Design review of the part built by this model. Coordinates are the model's own, in mm. Face numbers are marked on the shaded views. A direction names the side the tool comes from. Round coordinates to 2 decimals unless told otherwise and drop trailing zeros. Write each loop counter-clockwise with the first axis right and the second up, starting at its lowest first coordinate (ties: lowest second). Pieces come first, ordered by that corner, then holes. Notation, with made-up numbers: (13.5, 16) - (32.5, 16) arc R7 cw to (32.5, 26) - close; hole circle Ø8 at (-10, -24). An arc over 180 degrees is marked (long way). Use one line per item in the form item = value.
```python
from build123d import *

# Parameters (mm, degrees)
SKETCH1_W           = 2.8702
SKETCH1_H           = 3.5052
SKETCH2_R           = 1.7526
BOSS_EXTRUDE1_DEPTH = 7.9375
CUT_EXTRUDE1_DEPTH  = 1.6256
CHAMFER1_SIZE       = 0.47244
CHAMFER2_SIZE       = 0.3556
FILLET1_R           = 0.254


with BuildPart() as part:
    # Sketch1 → Revolve1 (revolve)
    with BuildSketch(Plane.XY):
        with Locations((1.4351, 1.7526)):
            Rectangle(SKETCH1_W, SKETCH1_H)
    revolve(axis=Axis((0, 3.5052, 0), (0, -1, 0)))

    # Sketch2 → Boss-Extrude1 (add)
    with BuildSketch(Plane.XZ):
        Circle(SKETCH2_R)
    extrude(amount=BOSS_EXTRUDE1_DEPTH)

    # Sketch3 → Cut-Extrude1 (cut)
    with BuildSketch(Plane(origin=(0, 3.5052, 0), x_dir=(-1, 0, 0), z_dir=(0, 1, 0))):
        Polygon((-0.799225978, 1.3843), (-1.598451955, 0), (-0.799225978, -1.3843), (0.799225978, -1.3843), (1.598451955, 0), (0.799225978, 1.3843), align=None)
    extrude(amount=-CUT_EXTRUDE1_DEPTH, mode=Mode.SUBTRACT)

    # Sketch4 → Cut-Revolve1 (revolve, cut)
    with BuildSketch(Plane.XY):
        Polygon((1.3843, 1.8796), (0, 1.8796), (0, 1.080374022), align=None)
    revolve(axis=Axis((0, 1.879625, 0), (0, -1, 0)), mode=Mode.SUBTRACT)

    # Chamfer1
    chamfer1_edges = [part.edges().sort_by_distance(p)[0] for p in [
        (-1.7526, -7.9375, 0),
    ]]
    chamfer(chamfer1_edges, length=CHAMFER1_SIZE)

    # Chamfer2
    chamfer2_edges = [part.edges().sort_by_distance(p)[0] for p in [
        (-2.8702, 3.5052, 0),
    ]]
    chamfer(chamfer2_edges, length=CHAMFER2_SIZE)

    # Fillet1
    fillet1_edges = [part.edges().sort_by_distance(p)[0] for p in [
        (-1.7526, 0, 0),
    ]]
    fillet(fillet1_edges, radius=FILLET1_R)


solid = part.part
```
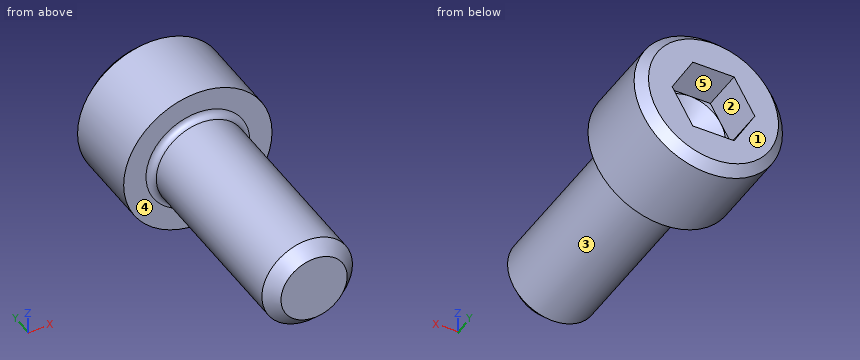
Q1. Draft analysis for pull direction X (two halves, no side actions). For the marked faces 3, 4 and 5, state which applies: released by +X, released by -X, zero draft, split by the parting line, or undercut.
Calculated:
face_3 = split by the parting line
face_4 = zero draft
face_5 = undercut
Q2. We need section B-B on y = -6. Write out the cut boundary in (x, z).
Calculated:
outline = circle Ø3.51 at (0, 0)
Q3. Machinability: for the marked faces 1 and 2, which of the approach directions +Z, -Z, +X, -X, +Y, -Y give a long, thin tool a straight path to every point of the face, cutting with its end or side? Answer none if there is none.
Calculated:
face_1 = +Z, -Z, +X, -X, +Y
face_2 = +Y
Q4. For P1, Ø2, axis at x = -0.5, y = -3.5, coming from the +Z side; P2, Ø1, axis at x = 1.5, z = 2.5, coming from the -Y side; P3, Ø0.6, axis at x = -0.5, z = -1, coming from the +Y side, all flat-tipped, find the tip position at first contact; note any pin that passes through.
Calculated:
P1 = 1.75
P2 = 0
P3 = 1.88
Q5. We need section A-A on y = 2.75. Write out the cut boundary in (x, z), then the cut area to 3 significant figures.
Calculated:
outline = circle Ø5.74 at (0, 0); hole (-1.6, 0) - (-0.8, -1.38) - (0.8, -1.38) - (1.6, 0) - (0.8, 1.38) - (-0.8, 1.38) - close
area = 19.2 mm2
Q6. To check wall thickness, follow line 1 along Y through (x, z) = (-1.55, 1.55); line 2 along Y through (x, z) = (-0.2, -1.15); line 3 along X through (y, z) = (1.25, -0.5). State the ranges of each line that lie inside material, in increasing order. Write a range as from..to.
Calculated:
line_1 = 0..3.51
line_2 = -7.94..1.75
line_3 = -2.83..2.83
